Geometry check sheet. Reference: drawing and pictorial views, mm from the part's lowest x, y, z. A direction names the side the tool comes from. Round coordinates to 2 decimals unless told otherwise and drop trailing zeros. Order: outer loops, then holes, each group sorted by start corner. A loop starts at its lowest first (then second) coordinate and runs counter-clockwise, first axis right, second up.
(1) Sectioned sample at D-D (z = 13). Record the boundary of the cut face in (x, y), plus the area to 3 significant figures.
(2) Sectioned sample at C-C (x = 15). Record the boundary of the cut face in (y, z).
(3) Set-up check for the marked faces 1 and 2: record each of +Z, -Z, +X, -X, +Y, -Y from which the full face is reachable in a straight line by a thin tool's end or side.
(4) Sectioned sample at A-A (x = 10.5). Record the boundary of the cut face in (y, z), plus the area to 3 significant figures.
(5) Sectioned sample at B-B (y = 2.5). Record the boundary of the cut face in (x, z), plus the area to 3 significant figures.
(6) Material ranges on line 1 along Z through (x, y) = (16.75, 15.5); line 2 along X through (y, z) = (14.5, 20.5); line 3 along Y through (x, z) = (26, 16.5), recorded low to high.
(7) Go/stop test with flat-tipped pins: pin 1 (1.5 mm diameter, centred on x = 7, z = 19, fed in from +Y); pin 2 (0.6 mm diameter, centred on x = 14.5, y = 31, fed in from -Z); pin 3 (1 mm diameter, centred on x = 15.5, y = 31, fed in from +Z). Record where each tip stops, or that it passes through.
(8) Release check for a two-part mould opening along Z. For the marked faces 3, 4, 5 and 6 record: +Z half, -Z half, draft (parallel to the pull), parting line (faces both ways), or undercut.
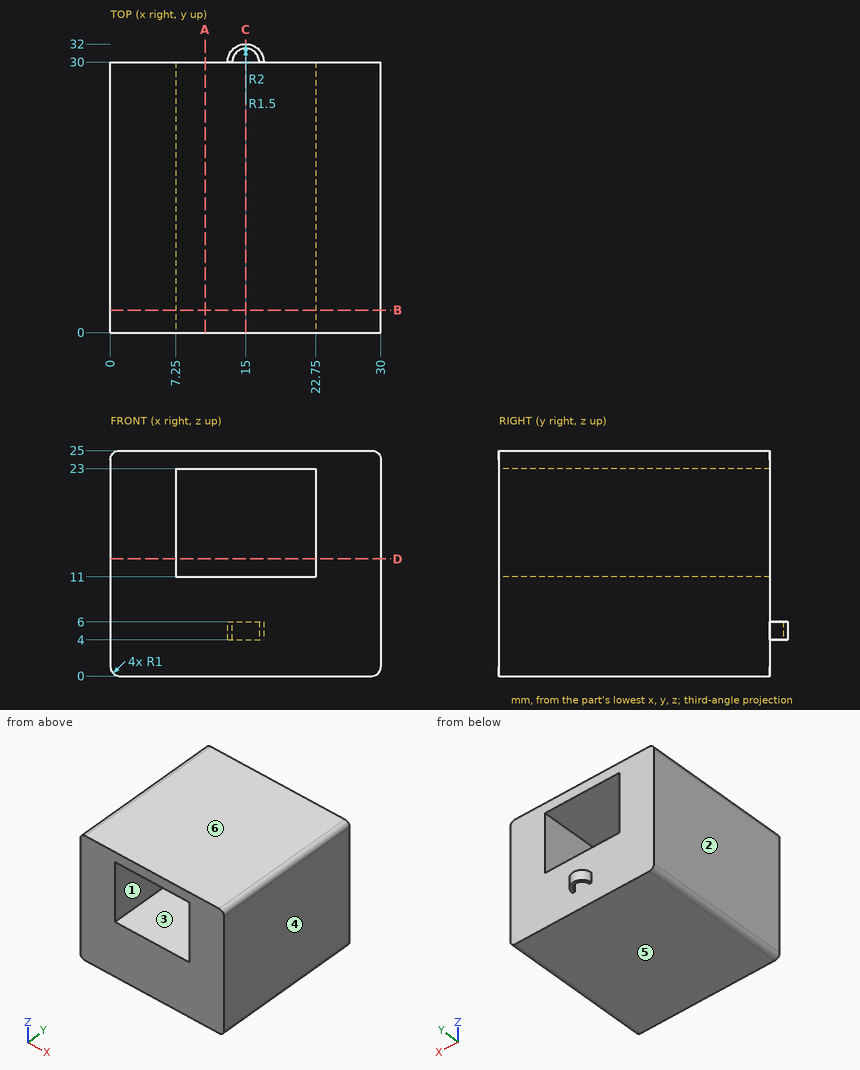
Answer below:
1. outline: (0, 0) - (7.25, 0) - (7.25, 30) - (0, 30) - close; (22.75, 0) - (30, 0) - (30, 30) - (22.75, 30) - close
1. area: 435 mm2
2. outline: (0, 0) - (30, 0) - (30, 11) - (0, 11) - close; (0, 23) - (30, 23) - (30, 25) - (0, 25) - close; (31.5, 4) - (32, 4) - (32, 6) - (31.5, 6) - close
3. face 1: +Y, -Y
3. face 2: +Z, -Z, -X, +Y, -Y
4. outline: (0, 0) - (30, 0) - (30, 11) - (0, 11) - close; (0, 23) - (30, 23) - (30, 25) - (0, 25) - close
4. area: 390 mm2
5. outline: (0, 1) arc R1 ccw to (1, 0) - (29, 0) arc R1 ccw to (30, 1) - (30, 24) arc R1 ccw to (29, 25) - (1, 25) arc R1 ccw to (0, 24) - close; hole (7.25, 11) - (22.75, 11) - (22.75, 23) - (7.25, 23) - close
5. area: 563 mm2
6. line 1: z = 0 to 11, 23 to 25
6. line 2: x = 0 to 7.25, 22.75 to 30
6. line 3: y = 0 to 30
7. pin 1: stops at y = 30
7. pin 2: passes through
7. pin 3: stops at z = 6
8. face 3: undercut
8. face 4: draft
8. face 5: -Z half
8. face 6: +Z half
